from build123d import *

# Parameters (mm, degrees)
F0_W     = 38.1
F0_H     = 444.5
F0_R     = 1.524
F0_W_2   = 3.302
F0_H_2   = 134.62
F0_R_2   = 2.159
F0_W_3   = 27.94
F0_H_3   = 22.098
F0_W_4   = 3.556
F0_H_4   = 6.096
F0_R_3   = 3.81
F0_W_5   = 18.542
F0_H_5   = 53.086
F0_R_4   = 1.905
F0_W_6   = 7.62
F0_H_6   = 34.798
F1_DEPTH = 3.175


with BuildPart() as f1:
    # F0 (on Top) → F1 (new body)
    with BuildSketch(Plane.XY):
        Rectangle(F0_W, F0_H)
        with Locations((-5.334, -124.714)):
            Circle(F0_R, mode=Mode.SUBTRACT)
        with Locations((-6.731, -53.594)):
            Rectangle(F0_W_2, F0_H_2, mode=Mode.SUBTRACT)
        with Locations((0, -217.297)):
            Circle(F0_R_2, mode=Mode.SUBTRACT)
        with Locations((0, -195.707)):
            Rectangle(F0_W_3, F0_H_3, mode=Mode.SUBTRACT)
        with Locations((0, -167.005)):
            Rectangle(F0_W_3, F0_H_3, mode=Mode.SUBTRACT)
        with Locations((0.762, -136.144)):
            Rectangle(F0_W_4, F0_H_4, mode=Mode.SUBTRACT)
        with Locations((8.89, -135.636)):
            Circle(F0_R_3, mode=Mode.SUBTRACT)
        with Locations((-5.334, 16.256)):
            Circle(F0_R, mode=Mode.SUBTRACT)
        with Locations((8.382, 33.528)):
            Circle(F0_R_3, mode=Mode.SUBTRACT)
        with Locations((3.302, 57.658)):
            Circle(F0_R_3, mode=Mode.SUBTRACT)
        with Locations((4.445, 110.617)):
            Rectangle(F0_W_5, F0_H_5, mode=Mode.SUBTRACT)
        with Locations((0, 217.551)):
            Circle(F0_R_2, mode=Mode.SUBTRACT)
        with Locations((10.287, 146.431)):
            Circle(F0_R_4, mode=Mode.SUBTRACT)
        with Locations((10.287, 154.051)):
            Circle(F0_R_4, mode=Mode.SUBTRACT)
        with Locations((9.906, 180.721)):
            Rectangle(F0_W_6, F0_H_6, mode=Mode.SUBTRACT)
    extrude(amount=F1_DEPTH)


solid = f1.part
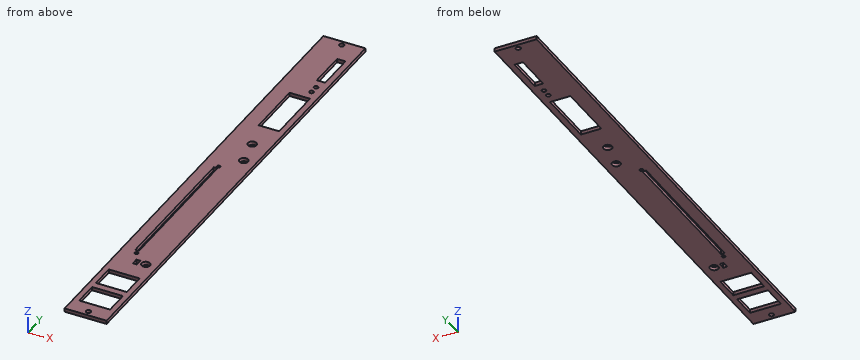
For this review, take the finished solid that the model builds, in its own axes (mm). Round coordinates to 2 decimals unless told otherwise and drop trailing zeros. Loops run counter-clockwise (first coordinate to the right, second up) from the corner with the lowest first, then second, coordinate; pieces in that order, holes last. Notation, with made-up numbers: (22.5, -35) - (30.5, -35) arc R31 ccw to (30.5, -5) - close; hole circle Ø6 at (60.5, 30.25). An arc over 180 degrees is marked (long way). Use one line per item in the form item = value.
Item 1: Clearance check with a flat-ended pin moving along its axis: P1, Ø5, axis at x = 9, y = 118, coming from the -Z side. State where the tip first meets the part, or that it passes through.
Answers:
P1 = through
Item 2: Consider section A-A on y = -57. Write out the cut boundary in (x, z) (3 decimals), then the cut area to 3 significant figures.
Answers:
outline = (-19.05, 0) - (-8.382, 0) - (-8.382, 3.175) - (-19.05, 3.175) - close; (-5.08, 0) - (19.05, 0) - (19.05, 3.175) - (-5.08, 3.175) - close
area = 110 mm^2
Item 3: Consider section B-B on z = 2.55. State how many separate pieces and enclosed holes the cut face has, then the cut area to 3 significant figures.
Answers:
separate_pieces = 1
enclosed_holes = 15
area = 13,800 mm^2
Item 4: For line 1 (Y direction, x = -5, z = 0.7); line 2 (Y direction, x = -12.5, z = 2.6); line 3 (X direction, y = -103.5, z = 0.85), list the stretches that pass through material, from the lowest coordinate up.
Answers:
line_1 = -222.25 to -206.76, -184.66 to -178.05, -155.96 to -126.2, -123.23 to 14.77, 17.74 to 222.25
line_2 = -222.25 to -206.76, -184.66 to -178.05, -155.96 to 222.25
line_3 = -19.05 to -8.38, -5.08 to 19.05
